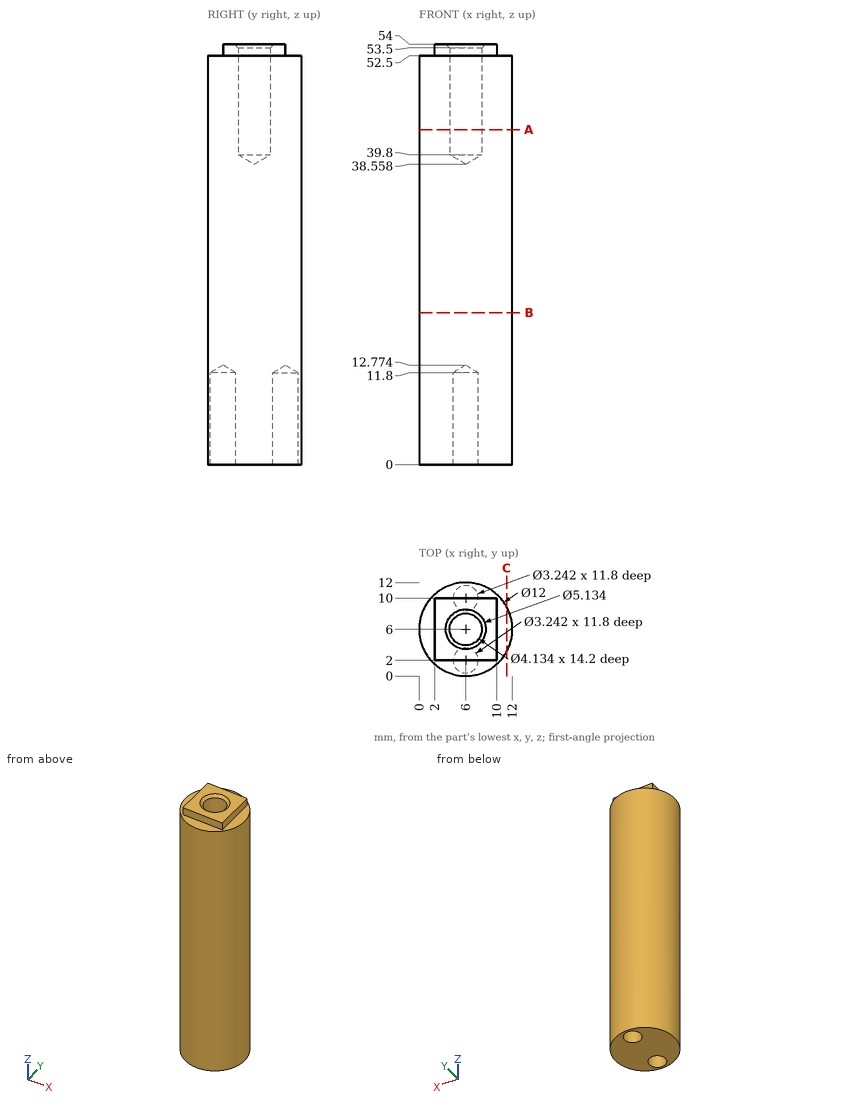
Geometry check sheet. Reference: drawing and pictorial views, mm from the part's lowest x, y, z. Give positions to 0.01 mm unless a question says otherwise; leave off trailing zeros. Order: outer loops, then holes, each group sorted by start corner. A loop starts at its lowest first (then second) coordinate and runs counter-clockwise, first axis right, second up. Notation, with made-up numbers: M 50,22.25 L 73,22.25 A30 cw 73,58.25 Z; hole C 34.25,32 d8. An arc over 180 degrees is marked long. Return JSON: item names as keys, results as strings. Group by question number.
1) Section check A-A on z = 43. Record the cut outline in (x, y).
2) Section check B-B on z = 19.5. Record the cut outline in (x, y).
3) Scan lines: line 1 (Y direction, x = 6, z = 45.75); line 2 (Z direction, x = 10.75, y = 5.5); line 3 (X direction, y = 2, z = 4.75). Record each from-to range of solid material in increasing order.
4) Section check C-C on x = 11.25. Record the cut outline in (y, z), and give its area (3 significant figures).
5) Go/stop test with flat-tipped pins: pin 1 Ø0.8 at (x, z) = (7.5, 53) entering from -Y; pin 2 Ø0.8 at (y, z) = (5, 53.5) entering from +X; pin 3 Ø3.5 at (x, y) = (6, 6) entering from -Z; pin 4 Ø1.2 at (y, z) = (4.5, 53.5) entering from -X. Record where each tip stops, or that it passes through.
Answer block:
{
 "1": {"outline": "C 6,6 d12; hole C 6,6 d4.13"},
 "2": {"outline": "C 6,6 d12"},
 "3": {"line 1": "y = 0 to 3.93, 8.07 to 12", "line 2": "z = 0 to 52.5", "line 3": "x = 1.53 to 4.38, 7.62 to 10.47"},
 "4": {"outline": "M 3.1,0 L 8.9,0 L 8.9,52.5 L 3.1,52.5 Z", "area": "305 mm^2"},
 "5": {"pin 1": "stops at y = 2", "pin 2": "stops at x = 10", "pin 3": "stops at z = 0", "pin 4": "stops at x = 2"}
}
